The listing builds one solid part. Answer for the finished solid, in the listing's coordinates (mm). Give positions to 0.01 mm unless a question says otherwise; leave off trailing zeros. Write each loop counter-clockwise with the first axis right and the second up, starting at its lowest first coordinate (ties: lowest second). Pieces come first, ordered by that corner, then holes. Notation, with made-up numbers: (41, 35.25) - (83, 35.25) arc R23 cw to (83, 57.25) - close; hole circle Ø8 at (80.5, 21). An arc over 180 degrees is marked (long way). One line per item, written item: value. Start each with the question number.
Solid Edge part; units mm, degrees
sketch "Sketch1" plane through (0, 0, 0) normal (0, -1, 0) x (1, 0, 0)
  circle A0 centre (0, 0) radius 10
  circle A1 centre (0, 0) radius 8
extrude "Protrusion1" add sketch "Sketch1" along normal mid plane 170
sketch "Sketch2" plane through (0, 0, 0) normal (0, 0, 1) x (1, 0, 0)
  circle A0 centre (0, -73) radius 2.5
  circle A1 centre (0, -58) radius 2.5
  circle A2 centre (0, 77) radius 2.5
  circle A3 centre (0, 62) radius 2.5
extrude "ExtrudedCutout_1" cut sketch "Sketch2" along normal mid plane 325.0188
properties material "PVC"
Item 1: The mould has two halves that part along X. Classify faces 1 (the cylindrical face through (2.31, -58.96, -8.78)), 2 (the cylindrical face through (2.31, -73.96, -8.78)), 3 (the flat face through (8.2, -85, 0)), 4 (the cylindrical face through (4.614, 1.19, 8.872)): +X half, -X half, draft (parallel to the pull), parting line (faces both ways), or undercut.
Item 2: Each of these flat-tipped pins is pushed along its axis until it touches: pin 1 Ø8 at (x, y) = (5.5, 64) entering from -Z; pin 2 Ø8 at (x, y) = (0, 62) entering from -Z; pin 3 Ø10 at (y, z) = (-52, 6) entering from +X; pin 4 Ø2 at (y, z) = (-12.5, -6) entering from +X. Where does it stop, or does it pass through?
Item 3: Find section B-B on z = 0. Determine the outline of the cut face in (x, y), plus the area to 3 significant figures.
Item 4: Straight lines are drawn through the part: line 1 along Y through (x, z) = (0, -8.85); line 2 along Y through (x, z) = (-0.5, 9); line 3 along X through (y, z) = (-39.5, 0.25). For each, find the intervals that lie inside material, in ascending order.
Item 5: Find section C-C on y = 15. Determine the outline of the cut face in (x, z), plus the area to 3 significant figures.
Item 6: Find section A-A on x = -4.25. Determine the outline of the cut face in (y, z), plus the area to 3 significant figures.
Values:
1. face 1: undercut
1. face 2: undercut
1. face 3: draft
1. face 4: parting line
2. pin 1: z = -9.89
2. pin 2: z = -10
2. pin 3: x = 9.95
2. pin 4: x = 8.66
3. outline: (-10, -85) - (-8, -85) - (-8, 85) - (-10, 85) - close; (8, -85) - (10, -85) - (10, 85) - (8, 85) - close
3. area: 680 mm^2
4. line 1: -85 to -75.5, -70.5 to -60.5, -55.5 to 59.5, 64.5 to 74.5, 79.5 to 85
4. line 2: -85 to -75.45, -70.55 to -60.45, -55.55 to 59.55, 64.45 to 74.55, 79.45 to 85
4. line 3: -10 to -8, 8 to 10
5. outline: circle Ø20 at (0, 0); hole circle Ø16 at (0, 0)
5. area: 113 mm^2
6. outline: (-85, -9.05) - (85, -9.05) - (85, -6.78) - (-85, -6.78) - close; (-85, 6.78) - (85, 6.78) - (85, 9.05) - (-85, 9.05) - close
6. area: 773 mm^2
